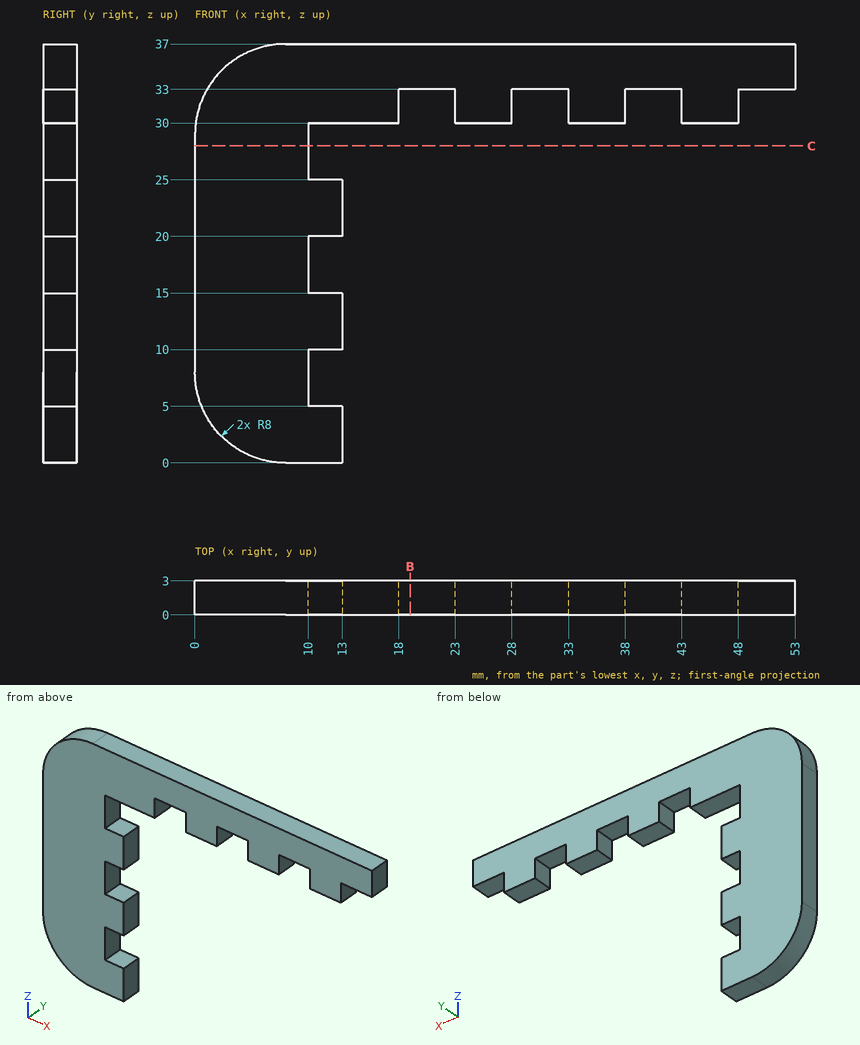
Input: dimensioned drawing with shaded views. Units: mm. Origin: part minimum x, y, z. Coordinates: 2 decimals unless noted, no trailing zeros. Order: outer loops, then holes, each group sorted by start corner. A loop starts at its lowest first (then second) coordinate and runs counter-clockwise, first axis right, second up.
(1) Material intervals for probe 1 along Z at (x, y) = (12, 0.75); probe 2 along X at (y, z) = (0.8, 31); probe 3 along Z at (x, y) = (19, 0.75), sorted ascending.
(2) Section query C-C (z = 28). Return the cut outline in (x, y).
(3) First-contact query: pin 1 (1 mm diameter, centred on x = 23.5, y = 1, fed in from -Z); pin 2 (1.5 mm diameter, centred on y = 2, z = 22, fed in from +X); pin 3 (0.9 mm diameter, centred on y = 1, z = 31.5, fed in from -X). Flat tips, straight axial feed; report the tip coordinate or a pass-through.
(4) Section query B-B (x = 19). Return the cut outline in (y, z).
Solution:
1. probe 1: z = 0 to 5, 10 to 15, 20 to 25, 30 to 37
1. probe 2: x = 0.25 to 18, 23 to 28, 33 to 38, 43 to 48
1. probe 3: z = 33 to 37
2. outline: (0, 0) - (10, 0) - (10, 3) - (0, 3) - close
3. pin 1: stops at z = 30
3. pin 2: stops at x = 13
3. pin 3: stops at x = 0.27
4. outline: (0, 33) - (3, 33) - (3, 37) - (0, 37) - close
